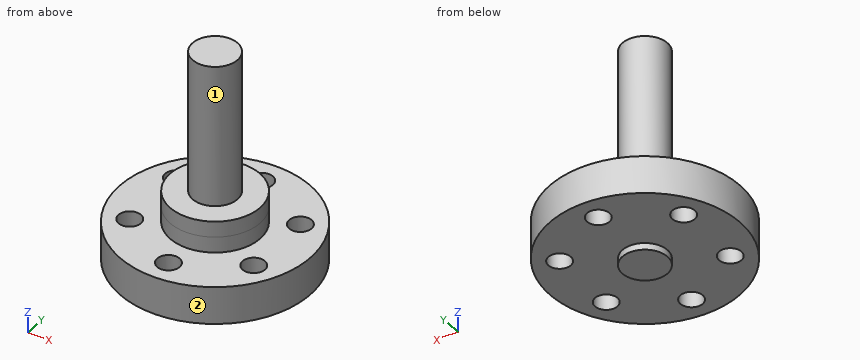
from build123d import *

# Parameters (mm, degrees)
SKETCH1_R           = 3
BOSS_EXTRUDE1_DEPTH = 29
SKETCH2_R           = 6
BOSS_EXTRUDE2_DEPTH = 2.1
SKETCH3_R           = 12.7
BOSS_EXTRUDE3_DEPTH = 5
SKETCH4_R           = 6
BOSS_EXTRUDE4_DEPTH = 2.1
SKETCH10_R          = 1.5
CUT_EXTRUDE1_DEPTH  = 10


with BuildPart() as part:
    # Sketch1 → Boss-Extrude1 (new body)
    with BuildSketch(Plane.XY):
        Circle(SKETCH1_R)
    extrude(amount=BOSS_EXTRUDE1_DEPTH)

    # Sketch2 → Boss-Extrude2 (add)
    with BuildSketch(Plane.XY.offset(8)):
        Circle(SKETCH2_R)
    extrude(amount=-BOSS_EXTRUDE2_DEPTH)

    # Sketch3 → Boss-Extrude3 (add)
    with BuildSketch(Plane(origin=(0, 0, 5.9), x_dir=(-1, 0, 0), z_dir=(0, 0, -1))):
        Circle(SKETCH3_R)
    extrude(amount=BOSS_EXTRUDE3_DEPTH)

    # Sketch4 → Boss-Extrude4 (add)
    with BuildSketch(Plane.XY.offset(8)):
        Circle(SKETCH4_R)
    extrude(amount=BOSS_EXTRUDE4_DEPTH)

    # Sketch10 → Cut-Extrude1 (cut)
    with BuildSketch(Plane(origin=(0, 0, 0.9), x_dir=(-1, 0, 0), z_dir=(0, 0, -1))):
        with Locations((8.227241336, 4.75)):
            Circle(SKETCH10_R)
        with Locations((0, 9.5)):
            Circle(SKETCH10_R)
        with Locations((8.227241336, -4.75)):
            Circle(SKETCH10_R)
        with Locations((0, -9.5)):
            Circle(SKETCH10_R)
        with Locations((-8.227241336, -4.75)):
            Circle(SKETCH10_R)
        with Locations((-8.227241336, 4.75)):
            Circle(SKETCH10_R)
    extrude(amount=-CUT_EXTRUDE1_DEPTH, mode=Mode.SUBTRACT)


solid = part.part
CAD build for the part. Positions are in the model's coordinates, mm. Face numbers are marked on the shaded views. A direction names the side the tool comes from. Give positions to 0.01 mm unless a question says otherwise; leave off trailing zeros. Write each loop counter-clockwise with the first axis right and the second up, starting at its lowest first coordinate (ties: lowest second). Pieces come first, ordered by that corner, then holes. Notation, with made-up numbers: M -11,10.5 L 20,10.5 A11 cw 20,22.5 Z; hole C 50.25,77.5 d1. An arc over 180 degrees is marked long. Put each result on its own line as item: value. Start each with the question number.
(1) Band-saw the part on C-C, the plane y = 4.75. Write the cut outline in (x, z).
(2) Band-saw the part on A-A, the plane x = 0. Write the cut outline in (y, z).
(3) Probe L1, parallel to Y at x = 0, z = 4.6; L2, parallel to Z at x = -0.5, y = -7; L3, parallel to X at y = -5.5, z = 3. List the from-to ranges inside material, lowest first.
(4) Band-saw the part on D-D, the plane z = 23. Write the cut outline in (x, y).
(5) Flat gauge pins, fed straight in: pin 1 Ø6 at (y, z) = (-2, 23) entering from -X; pin 2 Ø5 at (x, y) = (-8.23, -4.75) entering from -Z; pin 3 Ø3.5 at (x, y) = (8.23, -4.75) entering from +Z; pin 4 Ø2.5 at (x, y) = (8.23, 4.75) entering from -Z. Where does each tip first touch, or does it go through?
(6) Which spindle directions (+Z, -Z, +X, -X, +Y, -Y) get a long thin tool onto all of the face, cutting with end or side? Do the marked faces 1 and 2. Say none if no direction does.
(7) Band-saw the part on B-B, the plane y = 8.75. Write the cut outline in (x, z).
Response values:
1. outline: M -11.78,0.9 L -9.73,0.9 L -9.73,5.9 L -11.78,5.9 Z; M -6.73,0.9 L 6.73,0.9 L 6.73,5.9 L 3.67,5.9 L 3.67,10.1 L -3.67,10.1 L -3.67,5.9 L -6.73,5.9 Z; M 9.73,0.9 L 11.78,0.9 L 11.78,5.9 L 9.73,5.9 Z
2. outline: M -12.7,0.9 L -11,0.9 L -11,5.9 L -12.7,5.9 Z; M -8,0.9 L -3,0.9 L -3,0 L 3,0 L 3,0.9 L 8,0.9 L 8,5.9 L 6,5.9 L 6,10.1 L 3,10.1 L 3,29 L -3,29 L -3,10.1 L -6,10.1 L -6,5.9 L -8,5.9 Z; M 11,0.9 L 12.7,0.9 L 12.7,5.9 L 11,5.9 Z
3. L1: y = -12.7 to -11, -8 to 8, 11 to 12.7
3. L2: z = 0.9 to 5.9
3. L3: x = -11.45 to -9.53, -6.93 to 6.93, 9.53 to 11.45
4. outline: C 0,0 d6
5. pin 1: stops at x = -3
5. pin 2: stops at z = 0.9
5. pin 3: stops at z = 5.9
5. pin 4: passes through
6. face 1: +Z
6. face 2: +Z, -Z
7. outline: M -9.2,0.9 L -1.3,0.9 L -1.3,5.9 L -9.2,5.9 Z; M 1.3,0.9 L 9.2,0.9 L 9.2,5.9 L 1.3,5.9 Z
